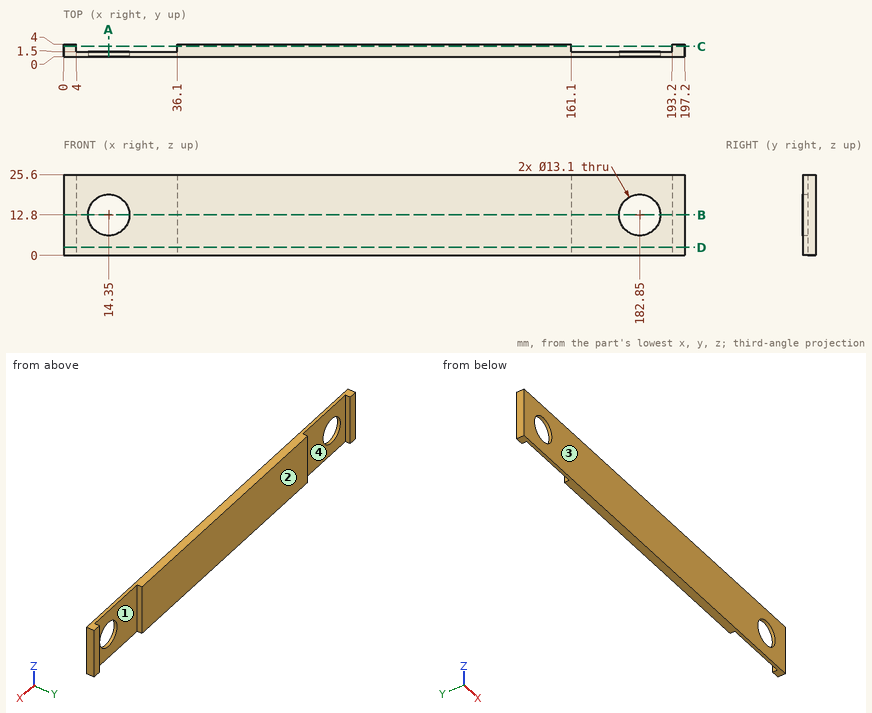
Verification items for this drawing (mm, ordinates from the low corner). A direction names the side the tool comes from. Round coordinates to 2 decimals unless told otherwise and drop trailing zeros. Write each loop counter-clockwise with the first axis right and the second up, starting at its lowest first coordinate (ties: lowest second). Pieces come first, ordered by that corner, then holes. Notation, with made-up numbers: M -26,0 L -7,0 A20 cw -7,36 Z; hole C -5.5,22.5 d1. An arc over 180 degrees is marked long. Write item = value, one per line. Start each with the question number.
1. Scan lines: line 1 (X direction, y = 1.55, z = 16.5); line 2 (X direction, y = 1.25, z = 12.8); line 3 (Y direction, x = 34.5, z = 20.75). Record each from-to range of solid material in increasing order. Write a range as [from, to].
2. Tool access check on the marked faces 1 and 2. Record the directions out of +Z, -Z, +X, -X, +Y, -Y that give a thin tool (end or side, any length) a straight path to the whole face; none if there is none.
3. Section check A-A, the plane x = 14.35. Record the cut outline in (y, z), then the cut area to 4 significant figures.
4. Section check C-C, the plane y = 3.25. Record the cut outline in (x, z).
5. Section check B-B, the plane z = 12.8. Record the cut outline in (x, y).
6. Gauge pin test, flat ends, axial feed: pin 1 (1.2 mm diameter, centred on y = 2.5, z = 8.5, fed in from -X); pin 2 (10.5 mm diameter, centred on x = 14.35, z = 12.8, fed in from -Y). Record the tip position at first contact, or that the pin passes through.
7. Release check for a two-part mould opening along X. For the marked faces 3 and 4 record: pulls with the +X half, pulls with the -X half, needs draft (parallel to the pull), parting line crosses it, or undercut.
8. Section check D-D, the plane z = 2.5. Record the cut outline in (x, y), then the cut area to 3 significant figures.
Results found:
q1.line_1 = [0, 4], [36.1, 161.1], [193.2, 197.2]
q1.line_2 = [0, 7.8], [20.9, 176.3], [189.4, 197.2]
q1.line_3 = [0, 1.5]
q2.face_1 = +Z, -Z, +Y
q2.face_2 = +Z, -Z, +X, -X, +Y
q3.outline = M 0,0 L 1.5,0 L 1.5,6.25 L 0,6.25 Z; M 0,19.35 L 1.5,19.35 L 1.5,25.6 L 0,25.6 Z
q3.area = 18.75 mm^2
q4.outline = M 0,0 L 4,0 L 4,25.6 L 0,25.6 Z; M 36.1,0 L 161.1,0 L 161.1,25.6 L 36.1,25.6 Z; M 193.2,0 L 197.2,0 L 197.2,25.6 L 193.2,25.6 Z
q5.outline = M 0,0 L 7.8,0 L 7.8,1.5 L 4,1.5 L 4,4 L 0,4 Z; M 20.9,0 L 176.3,0 L 176.3,1.5 L 161.1,1.5 L 161.1,4 L 36.1,4 L 36.1,1.5 L 20.9,1.5 Z; M 189.4,0 L 197.2,0 L 197.2,4 L 193.2,4 L 193.2,1.5 L 189.4,1.5 Z
q6.pin_1 = 0
q6.pin_2 = through
q7.face_3 = needs draft
q7.face_4 = undercut
q8.outline = M 0,0 L 197.2,0 L 197.2,4 L 193.2,4 L 193.2,1.5 L 161.1,1.5 L 161.1,4 L 36.1,4 L 36.1,1.5 L 4,1.5 L 4,4 L 0,4 Z
q8.area = 628 mm^2
